CAD build for the part. Positions are in the model's coordinates, mm. A direction names the side the tool comes from. Coordinates: 2 decimals unless noted, no trailing zeros. Loops run counter-clockwise (first coordinate to the right, second up) from the corner with the lowest first, then second, coordinate; pieces in that order, holes last. Notation, with made-up numbers: (58, 80) -> (116, 80) arc R30 ccw to (116, 119) -> close; hole circle Ø7 at (71, 74). An arc over 180 degrees is marked (long way). Write each question's results on one line, items separated by ' | '.
from build123d import *

# Parameters (mm, degrees)
SKETCH_1_W             = 40
SKETCH_1_H             = 40
EXTRUDE_637_DEPTH      = 8
SKETCH_2_W             = 28.8
SKETCH_2_H             = 29.8
CUT_EXTRUDE_819_DEPTH  = 5.3
SKETCH_3_W             = 28.8
SKETCH_3_H             = 20.86
CUT_EXTRUDE_1010_DEPTH = 29.776552955
SKETCH_4_W             = 12
SKETCH_4_H             = 4.47
CUT_EXTRUDE_1227_DEPTH = 2
SKETCH_5_W             = 28.8
SKETCH_5_H             = 0.5
EXTRUDE_1458_DEPTH     = 4
SKETCH_7_R             = 1.25
CUT_EXTRUDE_1697_DEPTH = 30.393876913
FILLET_1_R             = 2


with BuildPart() as part:
    # Эскиз1 → Extrude 637 (new body)
    with BuildSketch(Plane(origin=(0, 0, 0), x_dir=(1, 0, 0), z_dir=(0, 1, 0))):
        Rectangle(SKETCH_1_W, SKETCH_1_H)
    extrude(amount=EXTRUDE_637_DEPTH)

    # Эскиз2 → Cut-Extrude 819 (cut)
    with BuildSketch(Plane.XZ):
        Rectangle(SKETCH_2_W, SKETCH_2_H)
    extrude(amount=-CUT_EXTRUDE_819_DEPTH, mode=Mode.SUBTRACT)

    # Эскиз3 → Cut-Extrude 1010 (cut, through all)
    with BuildSketch(Plane.XZ.offset(-5.3)):
        Rectangle(SKETCH_3_W, SKETCH_3_H)
    extrude(amount=-CUT_EXTRUDE_1010_DEPTH, mode=Mode.SUBTRACT)

    # Эскиз4 → Cut-Extrude 1227 (cut)
    with BuildSketch(Plane.XZ.offset(-5.3)):
        with Locations((0, 12.665)):
            Rectangle(SKETCH_4_W, SKETCH_4_H)
        with Locations((0, -12.665)):
            Rectangle(SKETCH_4_W, SKETCH_4_H)
    extrude(amount=-CUT_EXTRUDE_1227_DEPTH, mode=Mode.SUBTRACT)

    # Эскиз5 → Extrude 1458 (add)
    with BuildSketch(Plane(origin=(0, 0, 10.43), x_dir=(-1, 0, 0), z_dir=(0, 0, -1))):
        with Locations((0, 7.75)):
            Rectangle(SKETCH_5_W, SKETCH_5_H)
    extrude(amount=EXTRUDE_1458_DEPTH)

    # Эскиз7 → Cut-Extrude 1697 (cut, through all)
    with BuildSketch(Plane.XZ):
        with Locations(Location((-16.5, 16.5, 0), (0, 0, 270))):
            Circle(SKETCH_7_R)
        with Locations(Location((16.5, 16.5, 0), (0, 0, 270))):
            Circle(SKETCH_7_R)
        with Locations(Location((16.5, -16.5, 0), (0, 0, 270))):
            Circle(SKETCH_7_R)
        with Locations(Location((-16.5, -16.5, 0), (0, 0, 270))):
            Circle(SKETCH_7_R)
    extrude(amount=-CUT_EXTRUDE_1697_DEPTH, mode=Mode.SUBTRACT)

    # Скругление1
    fillet_1_edges = [part.edges().sort_by_distance(p)[0] for p in [
        (20, 4, 20),
        (-20, 4, 20),
        (-20, 4, -20),
        (20, 4, -20),
    ]]
    fillet(fillet_1_edges, radius=FILLET_1_R)


solid = part.part
1) Slice it at A-A (x = -5). Write the cut outline in (y, z), then the cut area to 3 significant figures.
Outcome:
outline: (0, -20) -> (8, -20) -> (8, -10.43) -> (7.3, -10.43) -> (7.3, -14.9) -> (0, -14.9) -> close; (0, 14.9) -> (7.3, 14.9) -> (7.3, 10.43) -> (7.5, 10.43) -> (7.5, 6.43) -> (8, 6.43) -> (8, 20) -> (0, 20) -> close | area: 89.9 mm^2
2) Slice it at D-D (z = -1). Write the cut outline in (x, y).
Outcome:
outline: (-20, 0) -> (-14.4, 0) -> (-14.4, 8) -> (-20, 8) -> close; (14.4, 0) -> (20, 0) -> (20, 8) -> (14.4, 8) -> close
3) Slice it at B-B (y = 1.5). Write the cut outline in (x, z), then the cut area to 3 significant figures.
Outcome:
outline: (-20, -18) arc R2 ccw to (-18, -20) -> (18, -20) arc R2 ccw to (20, -18) -> (20, 18) arc R2 ccw to (18, 20) -> (-18, 20) arc R2 ccw to (-20, 18) -> close; hole circle Ø2.5 at (-16.5, -16.5); hole circle Ø2.5 at (-16.5, 16.5); hole (-14.4, -14.9) -> (14.4, -14.9) -> (14.4, 14.9) -> (-14.4, 14.9) -> close; hole circle Ø2.5 at (16.5, -16.5); hole circle Ø2.5 at (16.5, 16.5) | area: 719 mm^2
4) Drill centre lines: L1, parallel to X at y = 5.5, z = 16.5; L2, parallel to X at y = 4.5, z = 7.5; L3, parallel to Z at x = 5, y = 2.5. Where is each one in solid material? Low to high. Write a range as from..to.
Outcome:
L1: x = -20..-17.75, -15.25..15.25, 17.75..20 | L2: x = -20..-14.4, 14.4..20 | L3: z = -20..-14.9, 14.9..20
5) Two-plate mould, pull along Z, no slides. Class faces 1 (the cylindrical face through (17.554, 3.944, -17.172)), 2 (the flat face through (0, 4, -20)), 3 (the flat face through (0, 8, 9)): pulls with the +Z half, pulls with the -Z half, needs draft (parallel to the pull), parting line crosses it, or undercut.
Outcome:
face 1: undercut | face 2: pulls with the -Z half | face 3: needs draft
6) Pin check, flat tips, straight feed: pin 1 (2 mm diameter, centred on x = -15, z = 6.5, fed in from -Y); pin 2 (3.5 mm diameter, centred on x = 9, z = -12, fed in from -Y); pin 3 (1.5 mm diameter, centred on x = 16.5, z = 16.5, fed in from +Y). Stop position of each tip, or through.
Outcome:
pin 1: stops at y = 0 | pin 2: stops at y = 5.3 | pin 3: passes through
7) Slice it at C-C (x = 16.5). Write the cut outline in (y, z).
Outcome:
outline: (0, -20) -> (8, -20) -> (8, -17.75) -> (0, -17.75) -> close; (0, -15.25) -> (8, -15.25) -> (8, 15.25) -> (0, 15.25) -> close; (0, 17.75) -> (8, 17.75) -> (8, 20) -> (0, 20) -> close
8) Which spindle directions (+Z, -Z, +X, -X, +Y, -Y) get a long thin tool onto all of the face, cutting with end or side? Do faces 4 (the cylindrical face through (-19.43, 4.06, -19.4)), 5 (the flat face through (14.4, 4, 0)). Say none if no direction does.
Outcome:
face 4: -Z, -X, +Y, -Y | face 5: -Y
